```python
from build123d import *

# Parameters (mm, degrees)
CROQUIS1_R              = 4
CROQUIS1_R_2            = 1.5
SALIENTE_EXTRUIR1_DEPTH = 30
CROQUIS2_R              = 1.5
CORTAR_EXTRUIR1_DEPTH   = 30
REDONDEO1_R             = 0.5
REDONDEO2_R             = 0.5


with BuildPart() as part:
    # Croquis1 → Saliente-Extruir1 (new body)
    with BuildSketch(Plane.XY):
        with BuildLine():
            Line((-14.5, -15), (14.5, -15))
            ThreePointArc((14.5, -15), (14.853553391, -14.853553391), (15, -14.5))
            Line((15, -14.5), (15, 14.5))
            ThreePointArc((15, 14.5), (14.853553391, 14.853553391), (14.5, 15))
            Line((14.5, 15), (-14.5, 15))
            ThreePointArc((-14.5, 15), (-14.853553391, 14.853553391), (-15, 14.5))
            Line((-15, 14.5), (-15, -14.5))
            ThreePointArc((-15, -14.5), (-14.853553391, -14.853553391), (-14.5, -15))
        make_face()
        Circle(CROQUIS1_R, mode=Mode.SUBTRACT)
        with Locations((-7.45, 7.45)):
            Circle(CROQUIS1_R_2, mode=Mode.SUBTRACT)
        with Locations((7.45, 7.45)):
            Circle(CROQUIS1_R_2, mode=Mode.SUBTRACT)
        with Locations((-7.45, -7.45)):
            Circle(CROQUIS1_R_2, mode=Mode.SUBTRACT)
        with Locations((7.45, -7.45)):
            Circle(CROQUIS1_R_2, mode=Mode.SUBTRACT)
    extrude(amount=SALIENTE_EXTRUIR1_DEPTH)

    # Croquis2 → Cortar-Extruir1 (cut)
    with BuildSketch(Plane.XZ.offset(15)):
        with Locations((-12, 24.75)):
            Circle(CROQUIS2_R)
        with Locations((12, 24.75)):
            Circle(CROQUIS2_R)
        with Locations((12, 5.25)):
            Circle(CROQUIS2_R)
        with Locations((-12, 5.25)):
            Circle(CROQUIS2_R)
    extrude(amount=-CORTAR_EXTRUIR1_DEPTH, mode=Mode.SUBTRACT)

    # Redondeo1
    redondeo1_edges = [part.edges().sort_by_distance(p)[0] for p in [
        (15, 0, 30),
        (0, 15, 30),
        (-15, 0, 30),
        (0, -15, 30),
    ]]
    fillet(redondeo1_edges, radius=REDONDEO1_R)

    # Redondeo2
    redondeo2_edges = [part.edges().sort_by_distance(p)[0] for p in [
        (15, 0, 0),
        (0, -15, 0),
        (-15, 0, 0),
        (0, 15, 0),
    ]]
    fillet(redondeo2_edges, radius=REDONDEO2_R)


solid = part.part
```
Model file for the job. Use its own axes, mm. Coordinates: 2 decimals unless noted, no trailing zeros. Write each loop counter-clockwise with the first axis right and the second up, starting at its lowest first coordinate (ties: lowest second). Pieces come first, ordered by that corner, then holes. Notation, with made-up numbers: (-18.75, -7) - (7.25, -7) arc R21 ccw to (7.25, 22) - close; hole circle Ø2 at (80.25, 70). An arc over 180 degrees is marked (long way). One line per item, written item: value. Start each with the question number.
1. Slice it at C-C (y = 1.5). Write the cut outline in (x, z), plus the area to 3 significant figures.
2. Mould opens along Z. For faces 1 (the flat face through (0, -15, 15)), 2 (the cylindrical face through (11.805, -0.21, 26.237)), 3 (the flat face through (3, -3, 0)), 4 (the cylindrical face through (10.5, -0.2, 5.3)) say: released by +Z, released by -Z, zero draft, split by the parting line, or undercut.
3. Slice it at B-B (x = 0). Write the cut outline in (y, z), plus the area to 3 significant figures.
4. Probe line 1 (Z direction, x = 12, y = 5); line 2 (X direction, y = 8.5, z = 29); line 3 (X direction, y = 13, z = 5.75). List the from-to ranges inside material, lowest first. Write a range as from..to.
5. Slice it at D-D (y = 8). Write the cut outline in (x, z), plus the area to 3 significant figures.
6. Slice it at A-A (z = 5.25). Write the cut outline in (x, y).
Answers below:
1. outline: (-15, 0.5) arc R0.5 ccw to (-14.5, 0) - (-3.71, 0) - (-3.71, 30) - (-14.5, 30) arc R0.5 ccw to (-15, 29.5) - close; (3.71, 0) - (14.5, 0) arc R0.5 ccw to (15, 0.5) - (15, 29.5) arc R0.5 ccw to (14.5, 30) - (3.71, 30) - close; hole circle Ø3 at (-12, 5.25); hole circle Ø3 at (-12, 24.75); hole circle Ø3 at (12, 5.25); hole circle Ø3 at (12, 24.75)
1. area: 649 mm^2
2. face 1: zero draft
2. face 2: undercut
2. face 3: released by -Z
2. face 4: undercut
3. outline: (-15, 0.5) arc R0.5 ccw to (-14.5, 0) - (-4, 0) - (-4, 30) - (-14.5, 30) arc R0.5 ccw to (-15, 29.5) - close; (4, 0) - (14.5, 0) arc R0.5 ccw to (15, 0.5) - (15, 29.5) arc R0.5 ccw to (14.5, 30) - (4, 30) - close
3. area: 660 mm^2
4. line 1: z = 0..3.75, 6.75..23.25, 26.25..30
4. line 2: x = -15..-8.52, -6.38..6.38, 8.52..15
4. line 3: x = -15..-13.41, -10.59..10.59, 13.41..15
5. outline: (-15, 0.5) arc R0.5 ccw to (-14.5, 0) - (-8.85, 0) - (-8.85, 30) - (-14.5, 30) arc R0.5 ccw to (-15, 29.5) - close; (-6.05, 0) - (6.05, 0) - (6.05, 30) - (-6.05, 30) - close; (8.85, 0) - (14.5, 0) arc R0.5 ccw to (15, 0.5) - (15, 29.5) arc R0.5 ccw to (14.5, 30) - (8.85, 30) - close; hole circle Ø3 at (-12, 5.25); hole circle Ø3 at (-12, 24.75); hole circle Ø3 at (12, 5.25); hole circle Ø3 at (12, 24.75)
5. area: 704 mm^2
6. outline: (-15, -14.5) arc R0.5 ccw to (-14.5, -15) - (-13.5, -15) - (-13.5, 15) - (-14.5, 15) arc R0.5 ccw to (-15, 14.5) - close; (-10.5, -15) - (10.5, -15) - (10.5, 15) - (-10.5, 15) - close; (13.5, -15) - (14.5, -15) arc R0.5 ccw to (15, -14.5) - (15, 14.5) arc R0.5 ccw to (14.5, 15) - (13.5, 15) - close; hole circle Ø3 at (-7.45, -7.45); hole circle Ø3 at (-7.45, 7.45); hole circle Ø8 at (0, 0); hole circle Ø3 at (7.45, -7.45); hole circle Ø3 at (7.45, 7.45)
